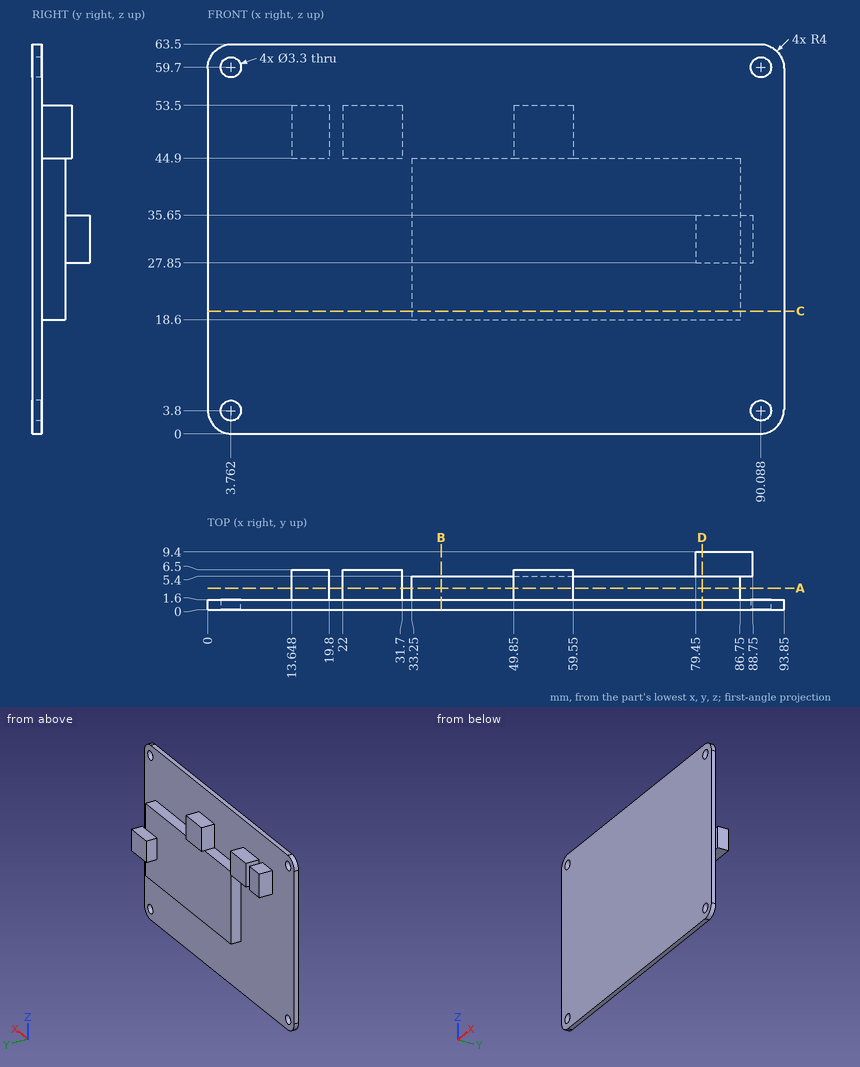
Source: three-view drawing plus pictorial views. Frame: mm from the lowest corner of the part. Coordinates: 2 decimals unless noted, no trailing zeros. Loops run counter-clockwise (first coordinate to the right, second up) from the corner with the lowest first, then second, coordinate; pieces in that order, holes last. Notation, with made-up numbers: (42.25, 89) -> (85.25, 89) arc R20 ccw to (85.25, 98) -> close; hole circle Ø10 at (63, -4.75). An arc over 180 degrees is marked (long way). Answer in a Markdown table with one row per item. Add a question column.
Q1. Section D-D on x = 80.5. Return the cut outline in (y, z).
Q2. Section C-C on z = 20. Return the cut outline in (x, y).
Q3. Section A-A on y = 3.5. Return the cut outline in (x, z).
Q4. Ray query, line 1 along X through (y, z) = (0.85, 59.7) (1 decimal); line 2 along X through (y, z) = (4.5, 52); line 3 along X through (y, z) = (8.25, 29.5). Return the intervals inside material, ascending.
Q5. Section B-B on x = 38. Return the cut outline in (y, z).
Q6. Contact query for flat-ended pins moving along their axis: pin 1 Ø1.9 at (y, z) = (3, 25.5) entering from +X; pin 2 Ø1.1 at (x, y) = (71, 3) entering from -Z; pin 3 Ø1.9 at (x, y) = (79, 3) entering from +Z; pin 4 Ø1.5 at (x, y) = (67, 6.5) entering from -Z. Output: stop coordinate, or through.
Computed values:
| question | item | result |
|---|---|---|
| 1 | outline | (0, 0) -> (1.6, 0) -> (1.6, 18.6) -> (5.4, 18.6) -> (5.4, 27.85) -> (9.4, 27.85) -> (9.4, 35.65) -> (5.4, 35.65) -> (5.4, 44.9) -> (1.6, 44.9) -> (1.6, 63.5) -> (0, 63.5) -> close |
| 2 | outline | (0, 0) -> (93.85, 0) -> (93.85, 1.6) -> (86.75, 1.6) -> (86.75, 5.4) -> (33.25, 5.4) -> (33.25, 1.6) -> (0, 1.6) -> close |
| 3 | outline | (13.65, 44.9) -> (19.8, 44.9) -> (19.8, 53.5) -> (13.65, 53.5) -> close; (22, 44.9) -> (31.7, 44.9) -> (31.7, 53.5) -> (22, 53.5) -> close; (33.25, 18.6) -> (86.75, 18.6) -> (86.75, 44.9) -> (59.55, 44.9) -> (59.55, 53.5) -> (49.85, 53.5) -> (49.85, 44.9) -> (33.25, 44.9) -> close |
| 4 | line 1 | x = 0 to 2.1, 5.4 to 88.4, 91.7 to 93.8 |
| 4 | line 2 | x = 13.65 to 19.8, 22 to 31.7, 49.85 to 59.55 |
| 4 | line 3 | x = 79.45 to 88.75 |
| 5 | outline | (0, 0) -> (1.6, 0) -> (1.6, 18.6) -> (5.4, 18.6) -> (5.4, 44.9) -> (1.6, 44.9) -> (1.6, 63.5) -> (0, 63.5) -> close |
| 6 | pin 1 | stops at x = 86.75 |
| 6 | pin 2 | stops at z = 18.6 |
| 6 | pin 3 | stops at z = 44.9 |
| 6 | pin 4 | passes through |
